Design review of the part built by this model. Coordinates are the model's own, in mm. A direction names the side the tool comes from. Give positions to 0.01 mm unless a question says otherwise; leave off trailing zeros. Loops run counter-clockwise (first coordinate to the right, second up) from the corner with the lowest first, then second, coordinate; pieces in that order, holes last. Notation, with made-up numbers: (-16.75, 4) - (23.25, 4) arc R11 ccw to (23.25, 12) - close; hole circle Ø2 at (6.5, 71.5). An arc over 180 degrees is marked (long way). Write each question's results on one line, items separated by ' | '.
```python
from build123d import *

# Parameters (mm, degrees)
SKETCH1_R           = 2.25
BOSS_EXTRUDE1_DEPTH = 20
SKETCH2_R           = 3.5
CUT_EXTRUDE1_DEPTH  = 62.660866844


with BuildPart() as part:
    # Sketch1 → Boss-Extrude1 (new body)
    with BuildSketch(Plane.XY):
        Polygon((-44.25, 0), (44.25, 0), (44.25, 6), (29.25, 6), (29.25, 44), (-29.25, 44), (-29.25, 6), (-44.25, 6), align=None)
        with Locations((24.815, 30.15)):
            Circle(SKETCH1_R, mode=Mode.SUBTRACT)
        with Locations(Location((24.815, 20.35, 0), (0, 0, 180))):
            Circle(SKETCH1_R, mode=Mode.SUBTRACT)
        with BuildLine():
            Line((-20.75, 35.5), (20.75, 35.5))
            Line((20.75, 35.5), (20.75, 15))
            Line((20.75, 15), (-20.75, 15))
            Line((-20.75, 15), (-20.75, 20.25))
            Line((-20.75, 20.25), (-22.567223321, 20.25))
            ThreePointArc((-22.567223321, 20.25), (-26.07307026, 18.484588726), (-25.75, 22.396527547))
            Line((-25.75, 22.396527547), (-25.75, 28.103472453))
            ThreePointArc((-25.75, 28.103472453), (-26.07307026, 32.015411274), (-22.567223321, 30.25))
            Line((-22.567223321, 30.25), (-20.75, 30.25))
            Line((-20.75, 30.25), (-20.75, 35.5))
        make_face(mode=Mode.SUBTRACT)
    extrude(amount=BOSS_EXTRUDE1_DEPTH)

    # Sketch2 → Cut-Extrude1 (cut, through all)
    with BuildSketch(Plane(origin=(0, 6, 0), x_dir=(1, 0, 0), z_dir=(0, 1, 0))):
        with Locations(Location((36.75, -10, 0), (0, 0, 180))):
            Circle(SKETCH2_R)
        with Locations((-36.75, -10)):
            Circle(SKETCH2_R)
    extrude(amount=-CUT_EXTRUDE1_DEPTH, mode=Mode.SUBTRACT)


solid = part.part
```
Item 1: We need section C-C on z = 4.5. Give the boundary of the cut face in (x, y) (3 decimals), then the cut area to 3 significant figures.
Output values:
outline: (-44.25, 0) - (44.25, 0) - (44.25, 6) - (29.25, 6) - (29.25, 44) - (-29.25, 44) - (-29.25, 6) - (-44.25, 6) - close; hole (-25.75, 22.397) arc R2.25 ccw (long way) to (-22.567, 20.25) - (-20.75, 20.25) - (-20.75, 15) - (20.75, 15) - (20.75, 35.5) - (-20.75, 35.5) - (-20.75, 30.25) - (-22.567, 30.25) arc R2.25 ccw (long way) to (-25.75, 28.103) - close; hole circle Ø4.5 at (24.815, 20.35); hole circle Ø4.5 at (24.815, 30.15) | area: 1,800 mm²
Item 2: Draft analysis for pull direction Z (two halves, no side actions). For faces 4 (the face through (20.75, 25, 10)), 5 (the face through (-39.527, 3.042, 12.13)), 6 (the face through (9, 13, 0)), state which applies: +Z half, -Z half, draft (parallel to the pull), parting line (faces both ways), or undercut.
Output values:
face 4: draft | face 5: undercut | face 6: -Z half
Item 3: Clearance check with flat-ended pins moving along their axes: P1, Ø6, axis at y = 25, z = 6.5, coming from the -X side; P2, Ø1.6, axis at y = 19, z = 7.5, coming from the +X side; P3, Ø6.5, axis at x = -36.75, z = 10, coming from the -Y side. State where each tip first meets the part, or that it passes through.
Output values:
P1: stops at x = -29.25 | P2: stops at x = 29.25 | P3: passes through
Item 4: Tool access review of faces 1 (the face through (40, 6, 8)), 2 (the face through (-44.25, 3, 10)), 3 (the face through (-22, 30.25, 10)): name each direction out of +Z, -Z, +X, -X, +Y, -Y from which nothing blocks a thin tool from reaching the whole face with its end or side.
Output values:
face 1: +Z, -Z, +X, +Y | face 2: +Z, -Z, -X, +Y, -Y | face 3: +Z, -Z
Item 5: We need section A-A on z = 10. Give the boundary of the cut face in (x, y) (3 decimals), then the cut area to 3 significant figures.
Output values:
outline: (-44.25, 0) - (-40.25, 0) - (-40.25, 6) - (-44.25, 6) - close; (-33.25, 0) - (33.25, 0) - (33.25, 6) - (29.25, 6) - (29.25, 44) - (-29.25, 44) - (-29.25, 6) - (-33.25, 6) - close; (40.25, 0) - (44.25, 0) - (44.25, 6) - (40.25, 6) - close; hole (-25.75, 22.397) arc R2.25 ccw (long way) to (-22.567, 20.25) - (-20.75, 20.25) - (-20.75, 15) - (20.75, 15) - (20.75, 35.5) - (-20.75, 35.5) - (-20.75, 30.25) - (-22.567, 30.25) arc R2.25 ccw (long way) to (-25.75, 28.103) - close; hole circle Ø4.5 at (24.815, 20.35); hole circle Ø4.5 at (24.815, 30.15) | area: 1,720 mm²
Item 6: We need section D-D on x = -36.75. Give the boundary of the cut face in (y, z), then the cut area to 3 significant figures.
Output values:
outline: (0, 0) - (6, 0) - (6, 6.5) - (0, 6.5) - close; (0, 13.5) - (6, 13.5) - (6, 20) - (0, 20) - close | area: 78.0 mm²
Item 7: Wall thickness on probe 1 along X at (y, z) = (20.35, 15.75) (3 decimals); probe 2 along Y at (x, z) = (10.5, 14.25); probe 3 along Z at (x, y) = (-36.75, 4.2): over which ranges is each line inside the solid? List them lowest first.
Output values:
probe 1: x = -29.25 to -27.065, 20.75 to 22.565, 27.065 to 29.25 | probe 2: y = 0 to 15, 35.5 to 44 | probe 3: z = 0 to 6.5, 13.5 to 20
Item 8: We need section B-B on x = 3.5. Give the boundary of the cut face in (y, z), then the cut area to 3 significant figures.
Output values:
outline: (0, 0) - (15, 0) - (15, 20) - (0, 20) - close; (35.5, 0) - (44, 0) - (44, 20) - (35.5, 20) - close | area: 470 mm²
